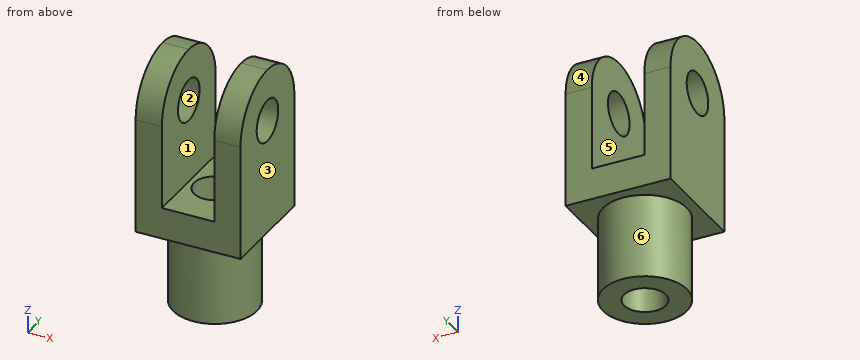
```python
from build123d import *

# Parameters (mm, degrees)
F1_DEPTH = 25
F2_R     = 20
F2_R_2   = 10
F3_DEPTH = 40
F4_DEPTH = 15
F5_R     = 10
F6_DEPTH = 56.6
F7_R     = 24.99999


# Not quite as in the source:
# - a fillet or chamfer is up to 0.001 mm smaller than in the source, because OpenCascade refuses the exact size


with BuildPart() as f1:
    # F0 (on Front) → F1 (new body, symmetric)
    with BuildSketch(Plane.XZ):
        Polygon((-12.5, 40), (-25, 40), (-25, -40), (25, -40), (25, 40), (12.5, 40), (12.5, -25), (-12.5, -25), align=None)
    extrude(amount=F1_DEPTH, both=True)

    # F2 (on face) → F3 (join)
    with BuildSketch(Plane(origin=(0, 0, -40), x_dir=(1, 0, 0), z_dir=(0, 0, -1))):
        Circle(F2_R)
        Circle(F2_R_2, mode=Mode.SUBTRACT)
    extrude(amount=F3_DEPTH)

    # F2 (on face) → F4 (cut)
    with BuildSketch(Plane(origin=(0, 0, -40), x_dir=(1, 0, 0), z_dir=(0, 0, -1))):
        Circle(F2_R_2)
    extrude(amount=-F4_DEPTH, mode=Mode.SUBTRACT)

    # F5 (on face) → F6 (cut)
    with BuildSketch(Plane(origin=(-25, 0, 0), x_dir=(0, -1, 0), z_dir=(-1, 0, 0))):
        with Locations((0, 15)):
            Circle(F5_R)
    extrude(amount=-F6_DEPTH, mode=Mode.SUBTRACT)

    # F7 (radius 25 in the source; OpenCascade refuses exactly that, so slightly less here)
    f7_edges = [f1.edges().sort_by_distance(p)[0] for p in [
        (18.75, 25, 40),
        (18.75, -25, 40),
        (-18.75, 25, 40),
        (-18.75, -25, 40),
    ]]
    fillet(f7_edges, radius=F7_R)


solid = f1.part
```
Input: part model. Units: mm. Frame: model coordinates. Face numbers are marked on the shaded views. A direction names the side the tool comes from. Give positions to 0.01 mm unless a question says otherwise; leave off trailing zeros. Order: outer loops, then holes, each group sorted by start corner. A loop starts at its lowest first (then second) coordinate and runs counter-clockwise, first axis right, second up. Notation, with made-up numbers: M 14.5,76 L 52.5,76 A16 cw 52.5,90 Z; hole C 16.5,5 d10. An arc over 180 degrees is marked long. Return JSON: item names as keys, results as strings.
1) Line query: L1, parallel to X at y = 0, z = -64; L2, parallel to X at y = 0, z = -22; L3, parallel to Y at x = 0, z = -34. Output: solid intervals per line, ascending. Write a range as [from, to].
Taken from the geometry:
{"L1": "x = [-20, -10], [10, 20]", "L2": "x = [-25, -12.5], [12.5, 25]", "L3": "y = [-25, -10], [10, 25]"}
2) Mould query, pull axis X, two halves, no side actions, for the marked faces 1, 2 and 3. Classes: released by +X, released by -X, zero draft, split by the parting line, or undercut.
Taken from the geometry:
{"face 1": "undercut", "face 2": "zero draft", "face 3": "released by +X"}
3) Section query D-D on z = -70. Output: boundary loops of the cut face in (x, y), and give its area (3 significant figures).
Taken from the geometry:
{"outline": "C 0,0 d40; hole C 0,0 d20", "area": "942 mm2"}
4) Contact query for flat-ended pins moving along their axis: pin 1 (2 mm diameter, centred on x = -12.5, z = -62.5, fed in from -Y); pin 2 (2 mm diameter, centred on x = 18, z = -44, fed in from -Y); pin 3 (3 mm diameter, centred on x = -10, y = -10.5, fed in from +Z); pin 4 (18 mm diameter, centred on y = 0, z = 15, fed in from +X). Output: stop coordinate, or through.
Taken from the geometry:
{"pin 1": "stops at y = -16.36", "pin 2": "stops at y = -10.54", "pin 3": "stops at z = -25", "pin 4": "passes through"}
5) Section query A-A on x = 0. Output: boundary loops of the cut face in (y, z), and give its area (3 significant figures).
Taken from the geometry:
{"outline": "M -25,-40 L -20,-40 L -20,-80 L -10,-80 L -10,-25 L -25,-25 Z; M 10,-80 L 20,-80 L 20,-40 L 25,-40 L 25,-25 L 10,-25 Z", "area": "1,250 mm2"}
6) Access query for the marked faces 4, 5 and 6. Directions: +Z, -Z, +X, -X, +Y, -Y. A direction counts if a zero-diameter tool reaches every point of the face in a straight line with its end or side. Return the directions, or none.
Taken from the geometry:
{"face 4": "+Z, +X, -X, +Y", "face 5": "+Z, +Y, -Y", "face 6": "-Z"}
7) Section query B-B on z = 22. Output: boundary loops of the cut face in (x, y), and give its area (3 significant figures).
Taken from the geometry:
{"outline": "M -25,-24 L -12.5,-24 L -12.5,-7.14 L -25,-7.14 Z; M -25,7.14 L -12.5,7.14 L -12.5,24 L -25,24 Z; M 12.5,-24 L 25,-24 L 25,-7.14 L 12.5,-7.14 Z; M 12.5,7.14 L 25,7.14 L 25,24 L 12.5,24 Z", "area": "843 mm2"}
